Autodesk Inventor part; units mm, degrees
ref_plane "YZ Plane" through (0, 0, 0) normal (1, 0, 0) x (0, 1, 0)
ref_plane "XZ Plane" through (0, 0, 0) normal (0, 1, 0) x (-1, 0, 0)
ref_plane "XY Plane" through (0, 0, 0) normal (0, 0, 1) x (1, 0, 0)
sketch "Boceto1" plane through (0, 0, 0) normal (0, 0, 1) x (1, 0, 0)
  line L0 (0, 0) -> (-50, 0)
  line L1 (-50, 0) -> (-50, 125)
  line L2 (0, 125) -> (0, 0)
  arc A0 (0, 125) -> (-50, 125) centre (-25, 125) ccw
  arc A1 (-20, 125) -> (-30, 125) centre (-25, 125) ccw
  line L3 (-25, 67.5) -> (-25, 60)
  arc A2 (-30, 60) -> (-20, 60) centre (-25, 60) ccw
  line L4 (-30, 60) -> (-30, 125)
  line L5 (-20, 60) -> (-20, 125)
  line L6 (0, 0) -> (-50, 0)
  line L7 (-50, 0) -> (-50, 38.1)
  line L8 (-50, 38.1) -> (0, 38.1)
  line L9 (0, 38.1) -> (0, 0)
  line L10 (-10, 28.1) -> (-40, 28.1)
  line L11 (-40, 28.1) -> (-40, 10)
  line L12 (-40, 10) -> (-10, 10)
  line L13 (-10, 10) -> (-10, 28.1)
  circle A3 centre (-40, 28.1) radius 2.5
  circle A4 centre (-10, 28.1) radius 2.5
  circle A5 centre (-40, 10) radius 2.5
  circle A6 centre (-10, 10) radius 2.5
  point P0 (-12.5, 10)
  point P1 (-10, 12.5)
  point P2 (-10, 25.6)
  point P3 (-12.5, 28.1)
  point P4 (-37.5, 28.1)
  point P5 (-40, 25.6)
  point P6 (-40, 12.5)
  point P7 (-37.5, 10)
  dimension "d2" = 10
  dimension "d3" = 65
  dimension "d4" = 10
  dimension "d5" = 38.1
  dimension "d6" = 10
  dimension "d7" = 5
  dimension "d8" = 5
  dimension "d9" = 5
  dimension "d10" = 5
extrude "Extrusión1" add sketch "Boceto1" along normal blind 3 contours L0 L1 L8 L2 | L8 L1 A0 L2 | L5 A2 L4 A1 | A3 L11 L10 | L10 L11 A3 | L10 A4 L13 A6 L12 A5 L11 A3 | A4 L13 L10 | L10 L13 A4 | A5 L12 L11 | L11 L12 A5 | A6 L12 L13 | L13 L12 A6
fillet "Empalme1" radius 2 2 edges at (0, 0, 1.5) (-50, 0, 1.5)
extrude "Extrusión2" cut sketch "Boceto1" along normal blind 3 contours L5 A2 L4 A1 | A3 L11 L10 | L10 L11 A3 | A4 L13 L10 | L10 L13 A4 | A5 L12 L11 | L11 L12 A5 | A6 L12 L13 | L13 L12 A6
Can you work these out from the model? Positions are in its coordinate system, mm. A direction names the side the tool comes from. Coordinates: 2 decimals unless noted, no trailing zeros. Loops run counter-clockwise (first coordinate to the right, second up) from the corner with the lowest first, then second, coordinate; pieces in that order, holes last. Notation, with made-up numbers: M 75,14 L 116,14 A16 ccw 116,21 Z; hole C -0.5,48 d2. An arc over 180 degrees is marked long. Answer as CSV lines item,"result". Start each with the question number.
1. For faces 4 (the face through (-25, 130, 1)), 5 (the face through (0, 64, 1)), which set-ups out of +Z, -Z, +X, -X, +Y, -Y let a thin tool reach every point of the face, with its end or its side?
2. Suppose I cut it at A-A, the plane y = 101. List the corners of the cut face in (x, z) for me.
3. Thinking about a two-plate mould opening in X: for faces 1 (the face through (-30, 92, 1)), 2 (the face through (-31, 76, 0)), 3 (the face through (-25.55, 149.994, 1.479)), which applies, +X half, -X half, draft (parallel to the pull), parting line (faces both ways), or undercut?
4. For pin 1 Ø1.5 at (y, z) = (130.5, 2.5) entering from +X; pin 2 Ø1.5 at (x, z) = (-17, 1) entering from +Y; pin 3 Ø4 at (x, y) = (-40, 10) entering from +Z, each with a flat end and sliding along its axis, tell me the tip position at first contact or that it passes through.
5. If I drill on probe 1 along X at (y, z) = (10, 2.2); probe 2 along X at (y, z) = (66, 0.65); probe 3 along Y at (x, z) = (-10, 1.95), over which ranges is the centre line in solid material (lowest first)? Write a range as [from, to].
6. Suppose I cut it at D-D, the plane x = -25. List the corners of the cut face in (y, z) for me.
7. Suppose I cut it at C-C, the plane z = 2.5. List the corners of the cut face in (x, y) for me.
8. Suppose I cut it at B-B, the plane y = 10. List the corners of the cut face in (x, z) for me, plus the area to 3 significant figures.
Output:
1,face 4,"+Z, -Z"
1,face 5,"+Z, -Z, +X, +Y, -Y"
2,outline,"M -50,0 L -30,0 L -30,3 L -50,3 Z; M -20,0 L 0,0 L 0,3 L -20,3 Z"
3,face 1,"undercut"
3,face 2,"draft"
3,face 3,"parting line"
4,pin 1,"stops at x = -0.46"
4,pin 2,"stops at y = 148.93"
4,pin 3,"passes through"
5,probe 1,"x = [-50, -42.5], [-37.5, -12.5], [-7.5, 0]"
5,probe 2,"x = [-50, -30], [-20, 0]"
5,probe 3,"y = [0, 7.5], [12.5, 25.6], [30.6, 145]"
6,outline,"M 0,0 L 55,0 L 55,3 L 0,3 Z; M 130,0 L 150,0 L 150,3 L 130,3 Z"
7,outline,"M -50,2 A2 ccw -48,0 L -2,0 A2 ccw 0,2 L 0,125 A25 ccw -50,125 Z; hole C -40,10 d5; hole C -40,28.1 d5; hole M -30,60 A5 ccw -20,60 L -20,125 A5 ccw -30,125 Z; hole C -10,10 d5; hole C -10,28.1 d5"
8,outline,"M -50,0 L -42.5,0 L -42.5,3 L -50,3 Z; M -37.5,0 L -12.5,0 L -12.5,3 L -37.5,3 Z; M -7.5,0 L 0,0 L 0,3 L -7.5,3 Z"
8,area,"120 mm^2"
